Geometry check sheet. Reference: the model listing, model coordinates, mm. Round coordinates to 2 decimals unless told otherwise and drop trailing zeros. Loops run counter-clockwise (first coordinate to the right, second up) from the corner with the lowest first, then second, coordinate; pieces in that order, holes last. Notation, with made-up numbers: M 32,-24.75 L 54,-24.75 A36 cw 54,12.25 Z; hole C 77.25,78 d1. An arc over 180 degrees is marked long. Write item = value, one per line.
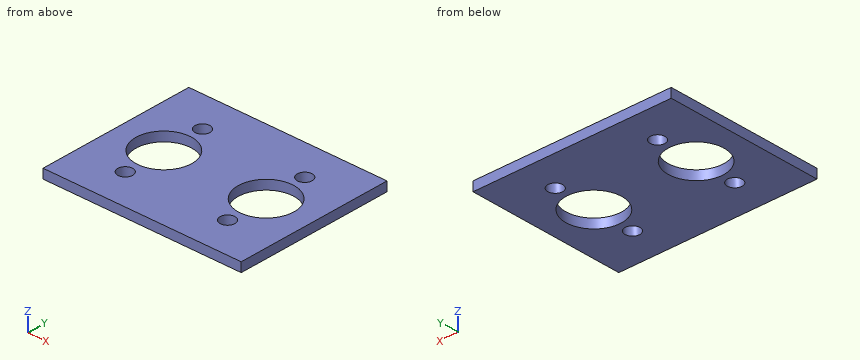
from build123d import *

# Parameters (mm, degrees)
SZKIC1_W                   = 106.6
SZKIC1_H                   = 85
ODGI_CIE_BAZOWE1_DEPTH     = 5
SZKIC6_R                   = 15
SZKIC6_R_2                 = 4
WYTNIJ_WYCI_GNI_CIE1_DEPTH = 69.353054065


# Sheet-metal steps are written as plain solids
with BuildPart() as part:
    # Szkic1 → Odgięcie bazowe1 (new body)
    with BuildSketch(Plane.XY):
        Rectangle(SZKIC1_W, SZKIC1_H)
    extrude(amount=-ODGI_CIE_BAZOWE1_DEPTH)

    # Szkic6 → Wytnij-wyciągnięcie1 (cut, through all)
    with BuildSketch(Plane.XY):
        with Locations((-27.5, 0)):
            Circle(SZKIC6_R)
        with Locations((27.5, 0)):
            Circle(SZKIC6_R)
        with Locations((-27.5, 22.5)):
            Circle(SZKIC6_R_2)
        with Locations((27.5, 22.5)):
            Circle(SZKIC6_R_2)
        with Locations((27.5, -22.5)):
            Circle(SZKIC6_R_2)
        with Locations((-27.5, -22.5)):
            Circle(SZKIC6_R_2)
    extrude(amount=-WYTNIJ_WYCI_GNI_CIE1_DEPTH, mode=Mode.SUBTRACT)


solid = part.part
(1) Sectioned sample at B-B on y = 0. Record the cut outline in (x, z), then the cut area to 3 significant figures.
Result set:
outline = M -53.3,-5 L -42.5,-5 L -42.5,0 L -53.3,0 Z; M -12.5,-5 L 12.5,-5 L 12.5,0 L -12.5,0 Z; M 42.5,-5 L 53.3,-5 L 53.3,0 L 42.5,0 Z
area = 233 mm2
(2) Sectioned sample at C-C on y = -22.5. Record the cut outline in (x, z), then the cut area to 3 significant figures.
Result set:
outline = M -53.3,-5 L -31.5,-5 L -31.5,0 L -53.3,0 Z; M -23.5,-5 L 23.5,-5 L 23.5,0 L -23.5,0 Z; M 31.5,-5 L 53.3,-5 L 53.3,0 L 31.5,0 Z
area = 453 mm2
(3) Sectioned sample at A-A on x = 27.5. Record the cut outline in (y, z).
Result set:
outline = M -42.5,-5 L -26.5,-5 L -26.5,0 L -42.5,0 Z; M -18.5,-5 L -15,-5 L -15,0 L -18.5,0 Z; M 15,-5 L 18.5,-5 L 18.5,0 L 15,0 Z; M 26.5,-5 L 42.5,-5 L 42.5,0 L 26.5,0 Z
(4) Material ranges on line 1 along Y through (x, z) = (-27.5, -3.55); line 2 along Y through (x, z) = (-26, -2.95); line 3 along X through (y, z) = (9, -4), recorded low to high. Write a range as from..to.
Result set:
line_1 = -42.5..-26.5, -18.5..-15, 15..18.5, 26.5..42.5
line_2 = -42.5..-26.21, -18.79..-14.92, 14.92..18.79, 26.21..42.5
line_3 = -53.3..-39.5, -15.5..15.5, 39.5..53.3
